Part print with two shaded views. Sizes in mm from the minimum x, y, z corner. A direction names the side the tool comes from. Round coordinates to 2 decimals unless told otherwise and drop trailing zeros. Order: outer loops, then holes, each group sorted by start corner. A loop starts at its lowest first (then second) coordinate and runs counter-clockwise, first axis right, second up. Notation, with made-up numbers: (8.25, 62) -> (45.25, 62) arc R7 cw to (45.25, 73) -> close; hole circle Ø11 at (7.25, 1.25). An arc over 180 degrees is marked (long way). Put each result on its own line as item: value. Start each with the question number.
Q1. Probe L1, parallel to Y at x = 8, z = 6; L2, parallel to X at y = 35, z = 4.5. List the from-to ranges inside material, lowest first.
Q2. Cut at C-C, the plane x = 5.5. List the corners of the cut face in (y, z).
Q3. Flat gauge pin, fed straight in: P1, Ø5, axis at x = 23.5, z = 7, coming from the -Y side. Where does the tip first touch, or does it go through?
Q4. Cut at A-A, the plane z = 2. List the corners of the cut face in (x, y).
Q5. 3-axis set-ups, long thin cutter, end or side, ignore diameter. For the marked faces 1 and 2: which of +Z, -Z, +X, -X, +Y, -Y reach the whole face in a straight line?
Q6. Cut at B-B, the plane y = 24.5. List the corners of the cut face in (x, z), and give its area (3 significant figures).
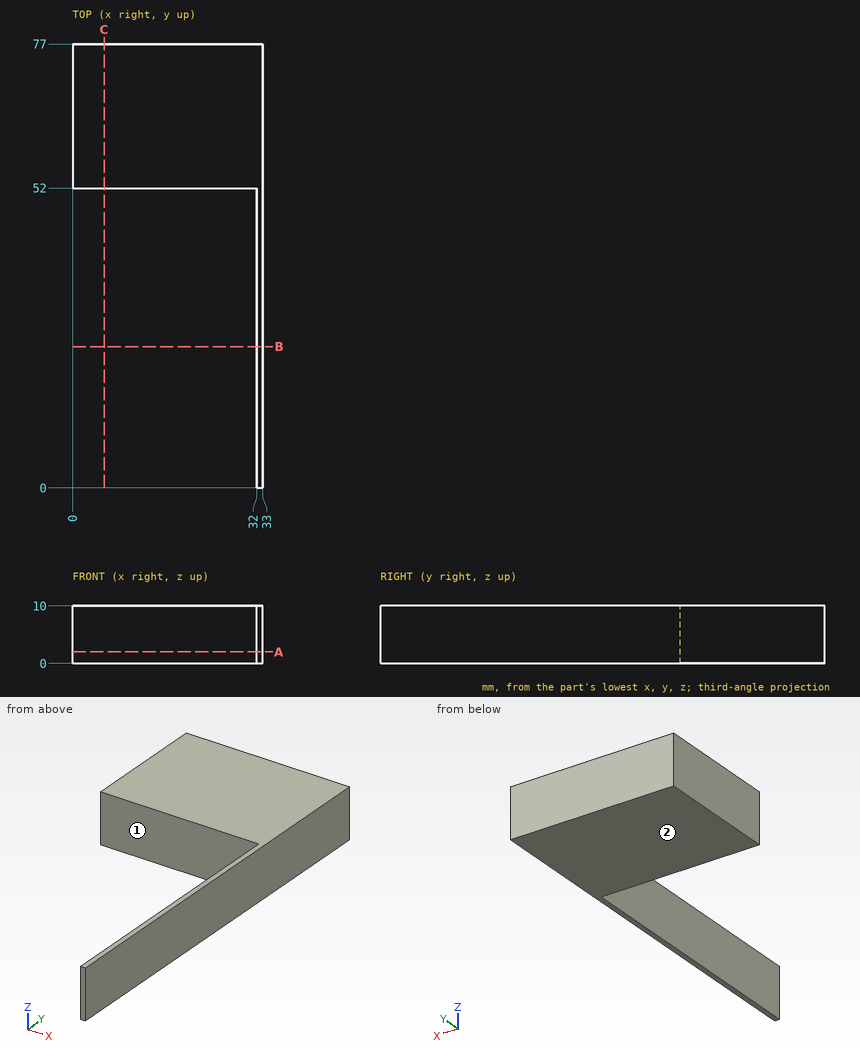
Ans:
1. L1: y = 52 to 77
1. L2: x = 32 to 33
2. outline: (52, 0) -> (77, 0) -> (77, 10) -> (52, 10) -> close
3. P1: stops at y = 52
4. outline: (0, 52) -> (32, 52) -> (32, 0) -> (33, 0) -> (33, 77) -> (0, 77) -> close
5. face 1: +Z, -Z, -X, -Y
5. face 2: -Z, +X, -X, +Y, -Y
6. outline: (32, 0) -> (33, 0) -> (33, 10) -> (32, 10) -> close
6. area: 10.0 mm^2
